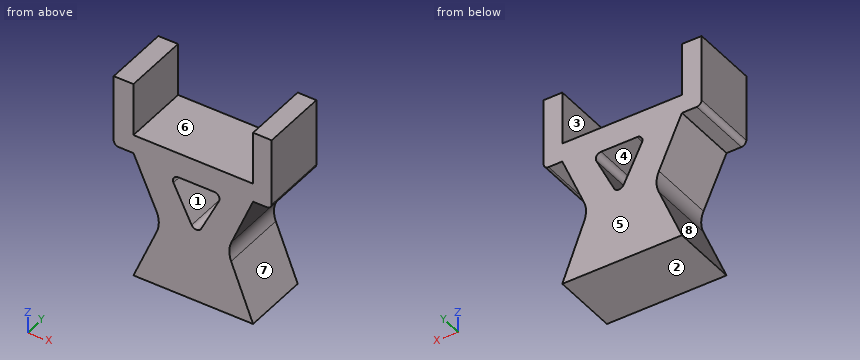
```python
from build123d import *

# Parameters (mm, degrees)
F0_W     = 45
F0_H     = 55
F1_DEPTH = 25
F3_DEPTH = 25
F5_DEPTH = 25
F7_DEPTH = 42.3


with BuildPart() as f1:
    # F0 (on Front) → F1 (new body)
    with BuildSketch(Plane.XZ):
        with Locations((-22.5, -99.278839)):
            Rectangle(F0_W, F0_H)
    extrude(amount=F1_DEPTH)

    # F2 (on face) → F3 (join)
    with BuildSketch(Plane.XZ.offset(25)):
        with BuildLine():
            Line((0, -51.778839), (0, -71.778839))
            Line((0, -71.778839), (0, -78.826934))
            Line((0, -78.826934), (5.137502, -78.826934))
            ThreePointArc((5.137502, -78.826934), (6.454487, -78.281421), (7, -76.964436))
            Line((7, -76.964436), (7, -51.826934))
            Line((7, -51.826934), (0, -51.778839))
        make_face()
        with BuildLine():
            Line((-45, -78.826934), (-45, -71.778839))
            Line((-45, -71.778839), (-45, -51.778839))
            Line((-45, -51.778839), (-52.44166, -51.826934))
            Line((-52.44166, -51.826934), (-52.44166, -76.964436))
            ThreePointArc((-52.44166, -76.964436), (-51.896147, -78.281421), (-50.579162, -78.826934))
            Line((-50.579162, -78.826934), (-45, -78.826934))
        make_face()
    extrude(amount=-F3_DEPTH)

    # F4 (on face) → F5 (cut)
    with BuildSketch(Plane.XZ.offset(25)):
        with BuildLine():
            Line((-8.242352, -105.71086), (0, -126.778839))
            Line((0, -126.778839), (0, -78.826934))
            Line((0, -78.826934), (-8.146975, -98.189167))
            ThreePointArc((-8.146975, -98.189167), (-8.928874, -101.940703), (-8.242352, -105.71086))
        make_face()
        with BuildLine():
            Line((-36.344591, -97.953365), (-45, -78.826934))
            Line((-45, -78.826934), (-45, -126.778839))
            Line((-45, -126.778839), (-36.23784, -105.954549))
            ThreePointArc((-36.23784, -105.954549), (-35.456027, -101.942814), (-36.344591, -97.953365))
        make_face()
    extrude(amount=-F5_DEPTH, mode=Mode.SUBTRACT)

    # F6 (on face) → F7 (cut)
    with BuildSketch(Plane.XZ.offset(25)):
        with BuildLine():
            ThreePointArc((-12.812875, -84.048576), (-12.911621, -82.110146), (-14.60875, -81.168331))
            Line((-14.60875, -81.168331), (-21.401127, -81.168331))
            Line((-21.401127, -81.168331), (-28.165059, -81.168331))
            ThreePointArc((-28.165059, -81.168331), (-29.866361, -82.116868), (-29.953914, -84.062758))
            Line((-29.953914, -84.062758), (-23.108318, -97.753949))
            ThreePointArc((-23.108318, -97.753949), (-21.311551, -98.859506), (-19.523588, -97.739767))
            Line((-19.523588, -97.739767), (-12.812875, -84.048576))
        make_face()
    extrude(amount=-F7_DEPTH, mode=Mode.SUBTRACT)


solid = f1.part
```
Check sheet for the modelled part. Datum: model origin and axes. Units: mm. Face numbers are marked on the shaded views. A direction names the side the tool comes from. Coordinates: 2 decimals unless noted, no trailing zeros. Loops run counter-clockwise (first coordinate to the right, second up) from the corner with the lowest first, then second, coordinate; pieces in that order, holes last. Notation, with made-up numbers: M 44.5,-19.75 L 84.5,-19.75 A18 cw 84.5,-15.75 Z; hole C 53,-2.5 d2. An arc over 180 degrees is marked long. Answer as a JSON object with one key per item and string values.
1. Sectioned sample at B-B on y = -2.25. Record the cut outline in (x, z) (1 decimal).
Outcome:
{"outline": "M -52.4,-77 A1.9 ccw -50.6,-78.8 L -45,-78.8 L -36.3,-98 A10 cw -36.2,-106 L -45,-126.8 L 0,-126.8 L -8.2,-105.7 A10 cw -8.1,-98.2 L 0,-78.8 L 5.1,-78.8 A1.9 ccw 7,-77 L 7,-51.8 L 0,-51.8 L 0,-71.8 L -45,-71.8 L -45,-51.8 L -52.4,-51.8 Z; hole M -30,-84.1 L -23.1,-97.8 A2 ccw -19.5,-97.7 L -12.8,-84 A2 ccw -14.6,-81.2 L -28.2,-81.2 A2 ccw Z"}
2. Release check for a two-part mould opening along Z. For the marked faces 1, 2 and 3 record: pulls with the +Z half, pulls with the -Z half, needs draft (parallel to the pull), parting line crosses it, or undercut.
Outcome:
{"face 1": "undercut", "face 2": "pulls with the -Z half", "face 3": "needs draft"}
3. Depth check by flat-ended pin: P1, Ø7.5, axis at x = -12.5, y = -10, coming from the +Z side; P2, Ø1, axis at y = -4, z = -99, coming from the +X side; P3, Ø4, axis at x = 2.5, y = -12, coming from the -Z side. Enter the tip coordinate at first touch or a pass-through.
Outcome:
{"P1": "z = -71.78", "P2": "x = -8.27", "P3": "z = -78.83"}
4. Sectioned sample at D-D on x = -34. Record the cut outline in (y, z), and give its area (4 significant figures).
Outcome:
{"outline": "M -25,-126.78 L 0,-126.78 L 0,-71.78 L -25,-71.78 Z", "area": "1,375 mm²"}
5. Sectioned sample at C-C on x = -25.5. Record the cut outline in (y, z).
Outcome:
{"outline": "M -25,-126.78 L 0,-126.78 L 0,-92.97 L -25,-92.97 Z; M -25,-81.17 L 0,-81.17 L 0,-71.78 L -25,-71.78 Z"}
6. Access from +Z, -Z, +X, -X, +Y, -Y to the whole of each face (thin tool, end or side, straight path). Record for the marked faces 4, 5, 6, 7 and 8.
Outcome:
{"face 4": "+Y, -Y", "face 5": "+Z, -Z, +X, -X, +Y", "face 6": "+Z, +Y, -Y", "face 7": "+X, +Y, -Y", "face 8": "-X, +Y, -Y"}
7. Scan lines: L1, parallel to X at y = -17, z = -56.5; L2, parallel to Z at x = -34, y = -12.75; L3, parallel to Z at x = -27, y = -18.5. Record each from-to range of solid material in increasing order. Write a range as from..to.
Outcome:
{"L1": "-52.44..-45, 0..7", "L2": "-126.78..-71.78", "L3": "-126.78..-89.97, -81.17..-71.78"}
8. Sectioned sample at A-A on z = -68. Record the cut outline in (x, y).
Outcome:
{"outline": "M -52.44,-25 L -45,-25 L -45,0 L -52.44,0 Z; M 0,-25 L 7,-25 L 7,0 L 0,0 Z"}
